Part print with two shaded views. Sizes in mm from the minimum x, y, z corner. A direction names the side the tool comes from. Give positions to 0.01 mm unless a question says otherwise; leave off trailing zeros. Order: outer loops, then holes, each group sorted by start corner. A loop starts at its lowest first (then second) coordinate and runs counter-clockwise, first axis right, second up. Notation, with made-up numbers: M 89.25,1 L 99.25,1 A15 ccw 99.25,19 Z; hole C 41,41 d9. An arc over 180 degrees is marked long. Return JSON: item names as keys, results as strings.
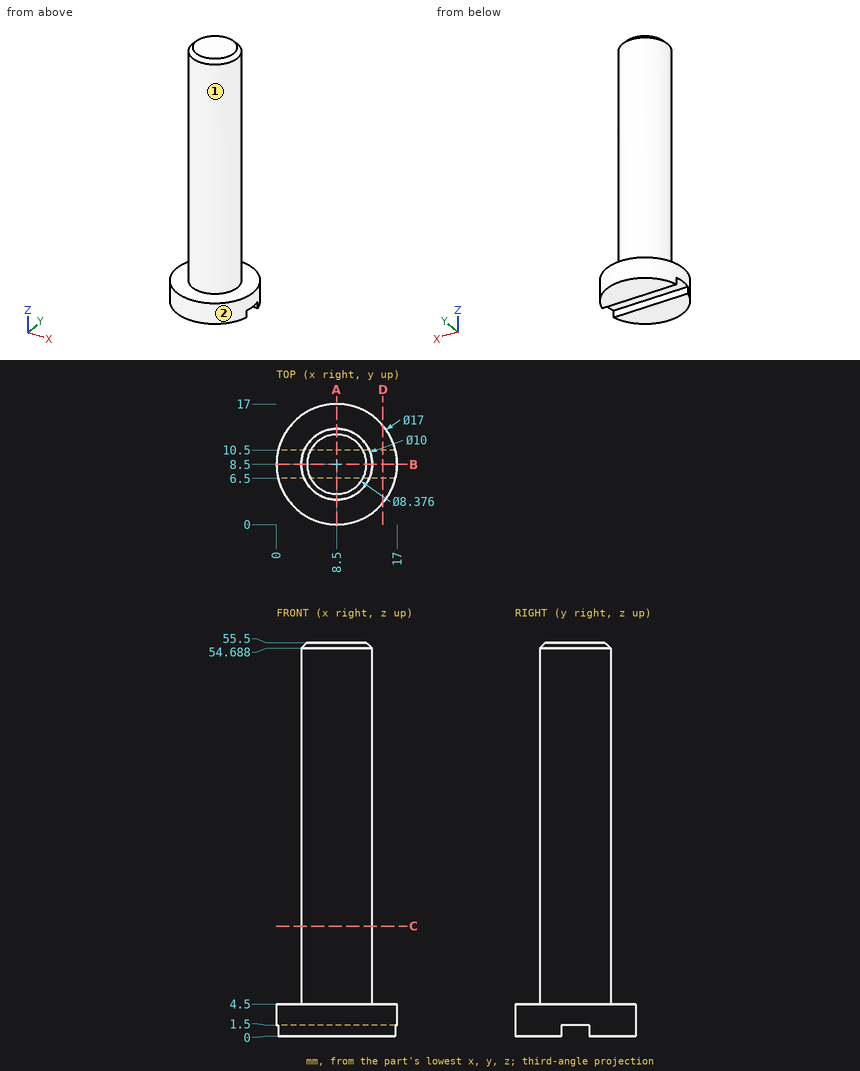
Q1. Pin check, flat tips, straight feed: pin 1 (3 mm diameter, centred on x = 3, z = 45.5, fed in from -Y); pin 2 (1.5 mm diameter, centred on x = 9.5, z = 41, fed in from -Y); pin 3 (0.8 mm diameter, centred on x = 9.5, z = 1, fed in from -Y). Stop position of each tip, or through.
Established:
{"pin 1": "stops at y = 5.5", "pin 2": "stops at y = 3.51", "pin 3": "stops at y = 0.02"}
Q2. Probe line 1 along Y through (x, z) = (8.75, 2.5); line 2 along X through (y, z) = (8.5, 6); line 3 along Z through (x, y) = (2.5, 4.75). List the from-to ranges inside material, lowest first.
Established:
{"line 1": "y = 0 to 17", "line 2": "x = 3.5 to 13.5", "line 3": "z = 0 to 4.5"}
Q3. 3-axis set-ups, long thin cutter, end or side, ignore diameter. For the marked faces 1 and 2: which of +Z, -Z, +X, -X, +Y, -Y reach the whole face in a straight line?
Established:
{"face 1": "+Z", "face 2": "+Z, -Z"}
Q4. Band-saw the part on A-A (x = 8.5). Give the cut face in (y, z).
Established:
{"outline": "M 0,0 L 6.5,0 L 6.5,1.5 L 10.5,1.5 L 10.5,0 L 17,0 L 17,4.5 L 13.5,4.5 L 13.5,54.69 L 12.69,55.5 L 4.31,55.5 L 3.5,54.69 L 3.5,4.5 L 0,4.5 Z"}
Q5. Band-saw the part on C-C (z = 15.5). Give the cut face in (x, y), then the cut area to 3 significant figures.
Established:
{"outline": "C 8.5,8.5 d10", "area": "78.5 mm²"}
Q6. Band-saw the part on D-D (x = 15). Give the cut face in (y, z), then the cut area to 3 significant figures.
Established:
{"outline": "M 3.02,0 L 6.5,0 L 6.5,1.5 L 10.5,1.5 L 10.5,0 L 13.98,0 L 13.98,4.5 L 3.02,4.5 Z", "area": "43.3 mm²"}
Q7. Band-saw the part on B-B (y = 8.5). Give the cut face in (x, z), then the cut area to 3 significant figures.
Established:
{"outline": "M 0,1.5 L 17,1.5 L 17,4.5 L 13.5,4.5 L 13.5,54.69 L 12.69,55.5 L 4.31,55.5 L 3.5,54.69 L 3.5,4.5 L 0,4.5 Z", "area": "560 mm²"}
